Autodesk Inventor part; units mm, degrees
ref_plane "Work Plane2" through (0, 0, 30) normal (1, 0, 0) x (0, 0, -1)
ref_plane "YZ Plane" through (0, 0, 0) normal (1, 0, 0) x (0, 1, 0)
ref_plane "XZ Plane" through (0, 0, 0) normal (0, 1, 0) x (-1, 0, 0)
sketch "Sketch1" plane through (0, 0, 0) normal (0, 1, 0) x (-1, 0, 0)
  line L0 (-34.5, 30) -> (34.5, 30)
  line L1 (34.5, 30) -> (34.5, -30)
  line L2 (34.5, -30) -> (-34.5, -30)
  line L3 (-34.5, -30) -> (-34.5, 30)
  line L4 (-34.5, 30) -> (34.5, -30) construction
  line L5 (34.5, 30) -> (-34.5, -30) construction
  point P0 (0, 0)
  dimension "d0" = 69
  dimension "d1" = 60
extrude "Extrusion1" add sketch "Sketch1" along normal blind 2
sketch "Sketch2" plane through (0, 2, 0) normal (0, 1, 0) x (1, 0, 0)
  line L0 (6.5, -15) -> (-6.5, -15)
  line L1 (-6.5, -15) -> (-6.5, 15)
  line L2 (-6.5, 15) -> (6.5, 15)
  line L3 (6.5, 15) -> (6.5, -15)
  line L4 (6.5, -15) -> (-6.5, 15) construction
  line L5 (-6.5, -15) -> (6.5, 15) construction
  line L6 (-24.5, -15) -> (-11.5, -15)
  line L7 (-11.5, -15) -> (-11.5, 15)
  line L8 (-11.5, 15) -> (-24.5, 15)
  line L9 (-24.5, 15) -> (-24.5, -15)
  line L10 (-24.5, -15) -> (-11.5, 15) construction
  line L11 (-11.5, -15) -> (-24.5, 15) construction
  line L12 (-24.5, 23) -> (-11.5, 23) construction
  line L13 (-11.5, 23) -> (-11.5, 16) construction
  line L14 (-11.5, 16) -> (-24.5, 16) construction
  line L15 (-24.5, 16) -> (-24.5, 23) construction
  line L16 (-6.5, 23) -> (6.5, 23) construction
  line L17 (6.5, 23) -> (6.5, 16) construction
  line L18 (6.5, 16) -> (-6.5, 16) construction
  line L19 (-6.5, 16) -> (-6.5, 23) construction
  line L20 (11.5, -15) -> (24.5, -15)
  line L21 (24.5, -15) -> (24.5, 15)
  line L22 (24.5, 15) -> (11.5, 15)
  line L23 (11.5, 15) -> (11.5, -15)
  line L24 (11.5, -15) -> (24.5, 15) construction
  line L25 (24.5, -15) -> (11.5, 15) construction
  line L26 (11.5, 23) -> (24.5, 23) construction
  line L27 (24.5, 23) -> (24.5, 16) construction
  line L28 (24.5, 16) -> (11.5, 16) construction
  line L29 (11.5, 16) -> (11.5, 23) construction
  circle A0 centre (32, -27.5) radius 1.55
  line L30 (-34.5, -30) -> (34.5, -30)
  line L31 (34.5, -30) -> (34.5, 30)
  circle A1 centre (32, 27.5) radius 1.55
  circle A2 centre (-32, 27.5) radius 1.55
  circle A3 centre (-32, -27.5) radius 1.55
  line L32 (34.5, 30) -> (-34.5, 30)
  line L33 (-34.5, 30) -> (-34.5, -30)
  line L34 (-15.8423, 16.4426) -> (-19.871, 16.4426)
  line L35 (-19.871, 16.4426) -> (-19.871, 17.5054)
  line L36 (-19.871, 17.5054) -> (-18.5858, 17.5054)
  line L37 (-18.5858, 17.5054) -> (-18.5858, 20.7333)
  line L38 (-18.5858, 20.7333) -> (-19.871, 20.7333)
  line L39 (-19.871, 20.7333) -> (-19.871, 21.7269)
  spline S0 degree 2 poles (-19.871, 21.7269) (-19.5893, 21.7269) (-19.0307, 21.8011) (-18.8626, 21.8802) knots 0 0 0 1 2 2 2
  spline S1 degree 2 poles (-18.8626, 21.8802) (-18.6698, 21.9791) (-18.4523, 22.3103) (-18.4325, 22.5574) knots 0 0 0 1 2 2 2
  line L40 (-18.4325, 22.5574) -> (-17.0979, 22.5574)
  line L41 (-17.0979, 22.5574) -> (-17.0979, 17.5054)
  line L42 (-17.0979, 17.5054) -> (-15.8423, 17.5054)
  line L43 (-15.8423, 17.5054) -> (-15.8423, 16.4426)
  line L44 (2.4296, 16.3907) -> (-2.0539, 16.3907)
  line L45 (-2.0539, 16.3907) -> (-2.0539, 17.3843)
  spline S2 degree 2 poles (-2.0539, 17.3843) (-1.4855, 17.8391) (-0.5759, 18.6399) (-0.2348, 19.0007) knots 0 0 0 1 2 2 2
  spline S3 degree 2 poles (-0.2348, 19.0007) (0.215, 19.4703) (0.6154, 20.1871) (0.6154, 20.5628) knots 0 0 0 1 2 2 2
  spline S4 degree 2 poles (0.6154, 20.5628) (0.6154, 20.9879) (0.1063, 21.4427) (-0.3485, 21.4427) knots 0 0 0 1 2 2 2
  spline S5 degree 2 poles (-0.3485, 21.4427) (-0.5808, 21.4427) (-0.9961, 21.329) (-1.2086, 21.24) knots 0 0 0 1 2 2 2
  spline S6 degree 2 poles (-1.2086, 21.24) (-1.4162, 21.1461) (-1.7128, 20.9484) (-1.787, 20.8989) knots 0 0 0 1 2 2 2
  line L46 (-1.787, 20.8989) -> (-1.9056, 20.8989)
  line L47 (-1.9056, 20.8989) -> (-1.9056, 22.2287)
  spline S7 degree 2 poles (-1.9056, 22.2287) (-1.6486, 22.3523) (-0.5512, 22.6093) (-0.042, 22.6093) knots 0 0 0 1 2 2 2
  spline S8 degree 2 poles (-0.042, 22.6093) (1.0455, 22.6093) (2.1627, 21.6404) (2.1627, 20.7655) knots 0 0 0 1 2 2 2
  spline S9 degree 2 poles (2.1627, 20.7655) (2.1627, 20.2267) (1.6535, 19.1886) (1.0653, 18.5954) knots 0 0 0 1 2 2 2
  spline S10 degree 2 poles (1.0653, 18.5954) (0.6945, 18.2296) (-0.0025, 17.6611) (-0.1557, 17.5425) knots 0 0 0 1 2 2 2
  line L48 (-0.1557, 17.5425) -> (2.4296, 17.5425)
  line L49 (2.4296, 17.5425) -> (2.4296, 16.3907)
  spline S11 degree 2 poles (20.2764, 18.2988) (20.2764, 17.8489) (19.9452, 17.1124) (19.6239, 16.8553) knots 0 0 0 1 2 2 2
  spline S12 degree 2 poles (19.6239, 16.8553) (19.3026, 16.5983) (18.4276, 16.3215) (17.7998, 16.3215) knots 0 0 0 1 2 2 2
  spline S13 degree 2 poles (17.7998, 16.3215) (17.088, 16.3215) (16.0697, 16.5588) (15.7483, 16.7071) knots 0 0 0 1 2 2 2
  line L50 (15.7483, 16.7071) -> (15.7483, 18.0318)
  line L51 (15.7483, 18.0318) -> (15.8966, 18.0318)
  spline S14 degree 2 poles (15.8966, 18.0318) (16.2328, 17.8193) (17.1374, 17.5029) (17.5131, 17.5029) knots 0 0 0 1 2 2 2
  spline S15 degree 2 poles (17.5131, 17.5029) (17.7355, 17.5029) (18.2546, 17.582) (18.4325, 17.7105) knots 0 0 0 1 2 2 2
  spline S16 degree 2 poles (18.4325, 17.7105) (18.5709, 17.8143) (18.739, 18.1159) (18.739, 18.3878) knots 0 0 0 1 2 2 2
  spline S17 degree 2 poles (18.739, 18.3878) (18.739, 18.6596) (18.5017, 18.9513) (18.304, 19.0205) knots 0 0 0 1 2 2 2
  spline S18 degree 2 poles (18.304, 19.0205) (18.1063, 19.0897) (17.5576, 19.1045) (17.345, 19.1045) knots 0 0 0 1 2 2 2
  line L52 (17.345, 19.1045) -> (17.083, 19.1045)
  line L53 (17.083, 19.1045) -> (17.083, 20.1772)
  line L54 (17.083, 20.1772) -> (17.3252, 20.1772)
  spline S19 degree 2 poles (17.3252, 20.1772) (17.6021, 20.1772) (18.0717, 20.2267) (18.2348, 20.3008) knots 0 0 0 1 2 2 2
  spline S20 degree 2 poles (18.2348, 20.3008) (18.3979, 20.3799) (18.5808, 20.6567) (18.5808, 20.894) knots 0 0 0 1 2 2 2
  spline S21 degree 2 poles (18.5808, 20.894) (18.5808, 21.0818) (18.4078, 21.3142) (18.2842, 21.3784) knots 0 0 0 1 2 2 2
  spline S22 degree 2 poles (18.2842, 21.3784) (18.1359, 21.4526) (17.7405, 21.502) (17.6021, 21.502) knots 0 0 0 1 2 2 2
  spline S23 degree 2 poles (17.6021, 21.502) (17.3796, 21.502) (16.91, 21.3982) (16.6925, 21.3142) knots 0 0 0 1 2 2 2
  spline S24 degree 2 poles (16.6925, 21.3142) (16.5195, 21.2499) (16.1438, 21.0423) (16.0548, 20.9879) knots 0 0 0 1 2 2 2
  line L55 (16.0548, 20.9879) -> (15.9263, 20.9879)
  line L56 (15.9263, 20.9879) -> (15.9263, 22.2929)
  spline S25 degree 2 poles (15.9263, 22.2929) (16.2427, 22.4264) (17.3104, 22.6785) (17.869, 22.6785) knots 0 0 0 1 2 2 2
  spline S26 degree 2 poles (17.869, 22.6785) (18.4128, 22.6785) (19.2136, 22.4907) (19.4953, 22.3078) knots 0 0 0 1 2 2 2
  spline S27 degree 2 poles (19.4953, 22.3078) (19.8068, 22.115) (20.1182, 21.5218) (20.1182, 21.1511) knots 0 0 0 1 2 2 2
  spline S28 degree 2 poles (20.1182, 21.1511) (20.1182, 20.6271) (19.5151, 19.846) (19.0208, 19.7323) knots 0 0 0 1 2 2 2
  line L57 (19.0208, 19.7323) -> (19.0208, 19.673)
  spline S29 degree 2 poles (19.0208, 19.673) (19.2383, 19.6434) (19.6535, 19.4852) (19.8513, 19.3072) knots 0 0 0 1 2 2 2
  spline S30 degree 2 poles (19.8513, 19.3072) (20.0342, 19.149) (20.2764, 18.6448) (20.2764, 18.2988) knots 0 0 0 1 2 2 2
  point P0 (0, 0)
  point P1 (-18, 0)
  point P2 (18, 0)
  dimension "d4" = 13
  dimension "d5" = 30
  dimension "d8" = 5
  dimension "d9" = 1
  dimension "d10" = 8
  dimension "d13" = 5
  dimension "d15" = 3.1
  dimension "d16" = 2.5
  dimension "d17" = 2.5
  dimension "d18" = 2.5
  dimension "d19" = 2.5
extrude "Extrusion2" cut sketch "Sketch2" against normal blind 2 contours L0 L1 L2 L3 | L9 L8 L7 L6 | L23 L22 L21 L20 | A0 | A1 | A2 | A3 | L34 L35 L36 L37 L38 L39 S0 S1 L40 L41 L42 L43 | L44 L45 S2 S3 S4 S5 S6 L46 L47 S7 S8 S9 S10 L48 L49 | S11 S12 S13 L50 L51 S14 S15 S16 S17 S18 L52 L53 L54 S19 S20 S21 S22 S23 S24 L55 L56 S25 S26 S27 S28 L57 S29 S30
ref_plane "Work Plane2" through (0, 0, 30) normal (1, 0, 0) x (0, 0, -1)
equation "\"d4\" = switch_len_at_clip"
equation "\"d5\" = switch_width_at_clip"
equation "\"switch_len_at_clip\" = 13"
equation "\"switch_width_at_clip\" = 30"
equation "\"pannel_height\" = 1"
properties part number "panel_switches"
Input: part model. Units: mm. Frame: model coordinates. A direction names the side the tool comes from. Coordinates: 2 decimals unless noted, no trailing zeros. Loops run counter-clockwise (first coordinate to the right, second up) from the corner with the lowest first, then second, coordinate; pieces in that order, holes last.
Q1. Section C-C, the plane x = -32. Return the cut outline in (y, z).
Results are:
outline: (0, -30) - (2, -30) - (2, -29.05) - (0, -29.05) - close; (0, -25.95) - (2, -25.95) - (2, 25.95) - (0, 25.95) - close; (0, 29.05) - (2, 29.05) - (2, 30) - (0, 30) - close
Q2. Contact query for a flat-ended pin moving along its axis: pin 1 (1 mm diameter, centred on x = -13, z = 11, fed in from +Y). Output: stop coordinate, or through.
Results are:
pin 1: passes through
Q3. Line query: line 1 along X through (y, z) = (0.4, 9); line 2 along Z through (x, y) = (-32, 0.9); line 3 along Z through (x, y) = (-22, 1). Output: solid intervals per line, ascending.
Results are:
line 1: x = -34.5 to -24.5, -11.5 to -6.5, 6.5 to 11.5, 24.5 to 34.5
line 2: z = -30 to -29.05, -25.95 to 25.95, 29.05 to 30
line 3: z = -30 to -15, 15 to 30
Q4. Mould query, pull axis X, two halves, no side actions, for faces 1 (the cylindrical face through (-31.17, 1.01, 26.19)), 2 (the flat face through (0, 1, 30)), 3 (the flat face through (34.5, 1, 0)), 4 (the flat face through (-34.5, 1, 0)). Classes: +X half, -X half, draft (parallel to the pull), parting line (faces both ways), or undercut.
Results are:
face 1: undercut
face 2: draft
face 3: +X half
face 4: -X half
Q5. Section A-A, the plane x = 15. Return the cut outline in (y, z).
Results are:
outline: (0, -30) - (2, -30) - (2, -15) - (0, -15) - close; (0, 15) - (2, 15) - (2, 30) - (0, 30) - close
Q6. Section D-D, the plane z = -27.5. Return the cut outline in (x, y).
Results are:
outline: (-34.5, 0) - (-33.55, 0) - (-33.55, 2) - (-34.5, 2) - close; (-30.45, 0) - (30.45, 0) - (30.45, 2) - (-30.45, 2) - close; (33.55, 0) - (34.5, 0) - (34.5, 2) - (33.55, 2) - close
Q7. Section B-B, the plane z = -3. Return the cut outline in (x, y).
Results are:
outline: (-34.5, 0) - (-24.5, 0) - (-24.5, 2) - (-34.5, 2) - close; (-11.5, 0) - (-6.5, 0) - (-6.5, 2) - (-11.5, 2) - close; (6.5, 0) - (11.5, 0) - (11.5, 2) - (6.5, 2) - close; (24.5, 0) - (34.5, 0) - (34.5, 2) - (24.5, 2) - close
Q8. Set-up query: faces 5 (the flat face through (24.5, 1, 0)), 6 (the flat face through (-7, 0, 0)). Return all of +Z, -Z, +X, -X, +Y, -Y with unobstructed straight access to the full face (end or side cutting, diameter ignored); none if empty.
Results are:
face 5: +Y, -Y
face 6: +Z, -Z, +X, -X, -Y
